```python
from build123d import *

# Parameters (mm, degrees)
F0_R      = 11.4
F0_R_2    = 10
F1_DEPTH  = 6.2
F2_R      = 13.6
F2_R_2    = 11.4
F3_DEPTH  = 1.4
F4_R      = 14.35
F4_R_2    = 11.4
F5_DEPTH  = 1.6
F6_R      = 12.8
F6_R_2    = 11.4
F7_DEPTH  = 1.5
F9_DEPTH  = 25
F10_R     = 0.9
F11_DEPTH = 1.5


with BuildPart() as f1:
    # F0 (on Top) → F1 (new body)
    with BuildSketch(Plane.XY):
        Circle(F0_R)
        Circle(F0_R_2, mode=Mode.SUBTRACT)
    extrude(amount=F1_DEPTH)

    # F2 (on face) → F3 (join)
    with BuildSketch(Plane.XY.offset(6.2)):
        Circle(F2_R)
        Circle(F2_R_2, mode=Mode.SUBTRACT)
    extrude(amount=-F3_DEPTH)

    # F4 (on face) → F5 (join)
    with BuildSketch(Plane(origin=(0, 0, 0), x_dir=(1, 0, 0), z_dir=(0, 0, -1))):
        Circle(F4_R)
        Circle(F4_R_2, mode=Mode.SUBTRACT)
    extrude(amount=-F5_DEPTH)

    # F6 (on face) → F7 (join)
    with BuildSketch(Plane.XY.offset(1.6)):
        Circle(F6_R)
        Circle(F6_R_2, mode=Mode.SUBTRACT)
    extrude(amount=F7_DEPTH)

    # F8 (on face) → F9 (cut)
    with BuildSketch(Plane.XY.offset(6.2)):
        with BuildLine():
            ThreePointArc((-3.85, 10.5174854409), (0, 11.2), (3.85, 10.5174854409))
            Line((3.85, 10.5174854409), (3.85, 11.2))
            Line((3.85, 11.2), (3.85, 13.0436766289))
            ThreePointArc((3.85, 13.0436766289), (0, 13.6), (-3.85, 13.0436766289))
            Line((-3.85, 13.0436766289), (-3.85, 11.2))
            Line((-3.85, 11.2), (-3.85, 10.5174854409))
        make_face()
        with BuildLine():
            ThreePointArc((-3.85, 13.0436766289), (0, 13.6), (3.85, 13.0436766289))
            Line((3.85, 13.0436766289), (3.85, 16.0734057426))
            Line((3.85, 16.0734057426), (-3.85, 16.0734057426))
            Line((-3.85, 16.0734057426), (-3.85, 13.0436766289))
        make_face()
        with BuildLine():
            ThreePointArc((-13.3865604245, -2.4), (-13.6, 0), (-13.3865604245, 2.4))
            Line((-13.3865604245, 2.4), (-16.2201337516, 2.4))
            Line((-16.2201337516, 2.4), (-16.2201337516, -2.4))
            Line((-16.2201337516, -2.4), (-13.3865604245, -2.4))
        make_face()
        with BuildLine():
            ThreePointArc((-10.9398354649, -2.4), (-11.2, 0), (-10.9398354649, 2.4))
            Line((-10.9398354649, 2.4), (-11.2, 2.4))
            Line((-11.2, 2.4), (-13.3865604245, 2.4))
            ThreePointArc((-13.3865604245, 2.4), (-13.6, 0), (-13.3865604245, -2.4))
            Line((-13.3865604245, -2.4), (-11.2, -2.4))
            Line((-11.2, -2.4), (-10.9398354649, -2.4))
        make_face()
        with BuildLine():
            ThreePointArc((10.9398354649, 2.4), (11.1347689066, 1.2070299898), (11.2, 0))
            ThreePointArc((11.2, 0), (11.1347689066, -1.2070299898), (10.9398354649, -2.4))
            Line((10.9398354649, -2.4), (11.2, -2.4))
            Line((11.2, -2.4), (13.3865604245, -2.4))
            ThreePointArc((13.3865604245, -2.4), (13.5465350141, -1.2047361176), (13.6, 0))
            ThreePointArc((13.6, 0), (13.5465350141, 1.2047361176), (13.3865604245, 2.4))
            Line((13.3865604245, 2.4), (11.2, 2.4))
            Line((11.2, 2.4), (10.9398354649, 2.4))
        make_face()
        with BuildLine():
            Line((16.2201337516, 2.4), (13.3865604245, 2.4))
            ThreePointArc((13.3865604245, 2.4), (13.5465350141, 1.2047361176), (13.6, 0))
            ThreePointArc((13.6, 0), (13.5465350141, -1.2047361176), (13.3865604245, -2.4))
            Line((13.3865604245, -2.4), (16.2201337516, -2.4))
            Line((16.2201337516, -2.4), (16.2201337516, 2.4))
        make_face()
        with BuildLine():
            Line((2.4, -11.2), (2.4, -10.9398354649))
            ThreePointArc((2.4, -10.9398354649), (0, -11.2), (-2.4, -10.9398354649))
            Line((-2.4, -10.9398354649), (-2.4, -11.2))
            Line((-2.4, -11.2), (-2.4, -13.3865604245))
            ThreePointArc((-2.4, -13.3865604245), (0, -13.6), (2.4, -13.3865604245))
            Line((2.4, -13.3865604245), (2.4, -11.2))
        make_face()
        with BuildLine():
            Line((2.4, -15.2210220695), (2.4, -13.3865604245))
            ThreePointArc((2.4, -13.3865604245), (0, -13.6), (-2.4, -13.3865604245))
            Line((-2.4, -13.3865604245), (-2.4, -15.2210220695))
            Line((-2.4, -15.2210220695), (2.4, -15.2210220695))
        make_face()
    extrude(amount=-F9_DEPTH, mode=Mode.SUBTRACT)

    # F10 (on face) → F11 (cut)
    with BuildSketch(Plane(origin=(0, 0, 0), x_dir=(1, 0, 0), z_dir=(0, 0, -1))):
        with BuildLine():
            ThreePointArc((-7.7090250609, 8.6090250609), (-8.2646099718, 9.4405166402), (-9.245421164, 9.245421164))
            Line((-9.245421164, 9.245421164), (-7.9726289579, 7.9726289579))
            ThreePointArc((-7.9726289579, 7.9726289579), (-7.7775334817, 8.2646099718), (-7.7090250609, 8.6090250609))
        make_face()
        with BuildLine():
            Line((-7.9726289579, 7.9726289579), (-9.245421164, 9.245421164))
            ThreePointArc((-9.245421164, 9.245421164), (-9.245421164, 7.9726289579), (-7.9726289579, 7.9726289579))
        make_face()
        with Locations((8.6090250609, 8.6090250609)):
            Circle(F10_R)
        with Locations((8.6090250609, -8.6090250609)):
            Circle(F10_R)
        with Locations((-8.6090250609, -8.6090250609)):
            Circle(F10_R)
    extrude(amount=-F11_DEPTH, mode=Mode.SUBTRACT)


solid = f1.part
```
Model file for the job. Use its own axes, mm. A direction names the side the tool comes from. Give positions to 0.01 mm unless a question says otherwise; leave off trailing zeros. Order: outer loops, then holes, each group sorted by start corner. A loop starts at its lowest first (then second) coordinate and runs counter-clockwise, first axis right, second up.
1) Mould opens along X. For faces 6 (the cylindrical face through (10.199, 8.997, 5.51)), 7 (the flat face through (8.6, -8.6, 1.5)), 8 (the flat face through (10, 9, 1.6)), 9 (the cylindrical face through (-8.8, 9.49, 0.74)) say: +X half, -X half, draft (parallel to the pull), parting line (faces both ways), or undercut.
2) Saw through at C-C, the plane y = 3.25. Write the cut outline in (x, z), then the cut area to 3 significant figures.
3) Saw through at A-A, the plane x = 0. Write the cut outline in (y, z), then the cut area to 3 significant figures.
4) Saw through at B-B, the plane z = 2.5. Write the cut outline in (x, y), then the cut area to 3 significant figures.
5) Pin check, flat tips, straight feed: pin 1 (2.5 mm diameter, centred on y = -13.5, z = 4.5, fed in from +X); pin 2 (0.5 mm diameter, centred on x = -8.5, y = -8.5, fed in from -Z); pin 3 (3 mm diameter, centred on x = 3, y = 7, fed in from +Z); pin 4 (3.5 mm diameter, centred on x = 12.5, z = 4.5, fed in from -Y). Stop position of each tip, or through.
6) Wall check: probe 1 along Z at (x, y) = (12.5, 4); probe 2 along Y at (x, z) = (0, 1.5); probe 3 along Y at (x, z) = (-3.25, 4). Give the ranges that are in metal, low to high.
7) 3-axis set-ups, long thin cutter, end or side, ignore diameter. For faces 1 (the flat face through (9, 8, 3.1)), 2 (the flat face through (-9, 8, 4.8)), 3 (the cylindrical face through (-8.125, -7.996, 3.938)), 4 (the flat face through (8, -9, 4.8)), 5 (the cylindrical face through (7.895, -8.061, 0.74)): which of +Z, -Z, +X, -X, +Y, -Y reach the whole face in a straight line?
8) Saw through at D-D, the plane y = 9. Write the cut outline in (x, z).
Computed:
1. face 6: +X half
1. face 7: undercut
1. face 8: draft
1. face 9: undercut
2. outline: (-13.98, 0) - (-9.46, 0) - (-9.46, 6.2) - (-13.21, 6.2) - (-13.21, 4.8) - (-10.93, 4.8) - (-10.93, 3.1) - (-12.38, 3.1) - (-12.38, 1.6) - (-13.98, 1.6) - close; (9.46, 0) - (13.98, 0) - (13.98, 1.6) - (12.38, 1.6) - (12.38, 3.1) - (10.93, 3.1) - (10.93, 4.8) - (13.21, 4.8) - (13.21, 6.2) - (9.46, 6.2) - close
2. area: 38.7 mm2
3. outline: (-11.2, 0) - (-10, 0) - (-10, 6.2) - (-11.2, 6.2) - close; (10, 0) - (11.2, 0) - (11.2, 6.2) - (10, 6.2) - close
3. area: 14.9 mm2
4. outline: (-12.57, -2.4) arc R12.8 ccw to (-2.4, -12.57) - (-2.4, -10.94) arc R11.2 ccw to (2.4, -10.94) - (2.4, -12.57) arc R12.8 ccw to (12.57, -2.4) - (10.94, -2.4) arc R11.2 ccw to (10.94, 2.4) - (12.57, 2.4) arc R12.8 ccw to (3.85, 12.21) - (3.85, 10.52) arc R11.2 ccw to (-3.85, 10.52) - (-3.85, 12.21) arc R12.8 ccw to (-12.57, 2.4) - (-10.94, 2.4) arc R11.2 ccw to (-10.94, -2.4) - close; hole circle Ø20 at (0, 0)
4. area: 165 mm2
5. pin 1: stops at x = 5.83
5. pin 2: stops at z = 1.5
5. pin 3: passes through
5. pin 4: stops at y = -8.3
6. probe 1: z = 0 to 1.6, 4.8 to 6.2
6. probe 2: y = -11.2 to -10, 10 to 11.2
6. probe 3: y = -10.93 to -9.46, 9.46 to 10.72
7. face 1: +X, +Y
7. face 2: -X, +Y
7. face 3: -X, -Y
7. face 4: +X, -Y
7. face 5: -Z
8. outline: (-11.18, 0) - (-9.42, 0) - (-9.42, 1.5) - (-7.8, 1.5) - (-7.8, 0) - (-4.36, 0) - (-4.36, 6.2) - (-10.2, 6.2) - (-10.2, 4.8) - (-7, 4.8) - (-7, 3.1) - (-9.1, 3.1) - (-9.1, 1.6) - (-11.18, 1.6) - close; (4.36, 0) - (7.8, 0) - (7.8, 1.5) - (9.42, 1.5) - (9.42, 0) - (11.18, 0) - (11.18, 1.6) - (9.1, 1.6) - (9.1, 3.1) - (7, 3.1) - (7, 4.8) - (10.2, 4.8) - (10.2, 6.2) - (4.36, 6.2) - close
